from build123d import *

# Parameters (mm, degrees)
SKETCH1_R           = 3
BOSS_EXTRUDE1_DEPTH = 1
SKETCH4_R           = 1.5
CUT_EXTRUDE1_DEPTH  = 5.5


with BuildPart() as part:
    # Sketch1 → Boss-Extrude1 (new body)
    with BuildSketch(Plane(origin=(0, 0, 0), x_dir=(1, 0, 0), z_dir=(0, 1, 0))):
        with Locations(Location((0, 0, 0), (0, 0, 270))):
            Circle(SKETCH1_R)
    extrude(amount=BOSS_EXTRUDE1_DEPTH)

    # Sketch3 → Revolve2 (revolve)
    with BuildSketch(Plane(origin=(0, 0, 0), x_dir=(0, 0, -1), z_dir=(1, 0, 0))):
        with BuildLine():
            Line((-1.156919819, 1), (0, 1))
            Line((0, 1), (0, 4))
            Line((0, 4), (0, 7))
            ThreePointArc((0, 7), (-2.121320344, 6.121320344), (-3, 4))
            ThreePointArc((-3, 4), (-2.823253346, 2.98548507), (-2.313839638, 2.090511553))
            Line((-2.313839638, 2.090511553), (-2.313839638, 1))
            Line((-2.313839638, 1), (-1.156919819, 1))
        make_face()
    revolve(axis=Axis((0, 4, 0), (0, 1, 0)))

    # Sketch4 → Cut-Extrude1 (cut)
    with BuildSketch(Plane.XZ):
        with Locations(Location((0, 0, 0), (0, 0, 270))):
            Circle(SKETCH4_R)
    extrude(amount=-CUT_EXTRUDE1_DEPTH, mode=Mode.SUBTRACT)


solid = part.part
Geometry check sheet. Reference: the model listing, model coordinates, mm. A direction names the side the tool comes from. Coordinates: 2 decimals unless noted, no trailing zeros. Order: outer loops, then holes, each group sorted by start corner. A loop starts at its lowest first (then second) coordinate and runs counter-clockwise, first axis right, second up. Notation, with made-up numbers: (39, 18) - (85, 18) arc R21 cw to (85, 56) - close; hole circle Ø7 at (-6, 88). An arc over 180 degrees is marked (long way). Answer in a Markdown table with one row per item. Add a question column.
1) Cross-section at A-A, the plane z = 0. Record the cut outline in (x, y), then the cut area to 3 significant figures.
2) Set-up check for faces 4 (the cylindrical face through (0.45, 2.71, -1.43)), 5 (the flat face through (-2, 1, 2)): record each of +Z, -Z, +X, -X, +Y, -Y from which the full face is reachable in a straight line by a thin tool's end or side.
3) Release check for a two-part mould opening along Y. For faces 1 (the cylindrical face through (0.9, 0.49, 2.86)), 2 (the flat face through (-1.3, 0, 1.3)), 3 (the cylindrical face through (-2.26, 1.54, -0.5)) record: +Y half, -Y half, draft (parallel to the pull), parting line (faces both ways), or undercut.
4) Cross-section at B-B, the plane x = 0. Record the cut outline in (y, z).
5) Cross-section at D-D, the plane y = 4.5. Record the cut outline in (x, z), then the cut area to 3 significant figures.
6) Gauge pin test, flat ends, axial feed: P1, Ø2, axis at x = 1, z = -0.5, coming from the +Y side; P2, Ø0.9, axis at x = 0, z = -0.5, coming from the -Y side; P3, Ø1, axis at y = 3.5, z = -2, coming from the -X side. Record the tip position at first contact, or that the pin passes through.
7) Material ranges on line 1 along X through (y, z) = (1.7, 0); line 2 along X through (y, z) = (0.5, 1.25); line 3 along Y through (x, z) = (1.65, 2.25), recorded low to high. Write a range as [from, to].
8) Cross-section at C-C, the plane x = -2.55. Record the cut outline in (y, z), then the cut area to 3 significant figures.
Check result:
| question | item | result |
|---|---|---|
| 1 | outline | (-3, 0) - (-1.5, 0) - (-1.5, 5.5) - (1.5, 5.5) - (1.5, 0) - (3, 0) - (3, 1) - (2.31, 1) - (2.31, 2.09) arc R3 ccw (long way) to (-2.31, 2.09) - (-2.31, 1) - (-3, 1) - close |
| 1 | area | 19.3 mm² |
| 2 | face 4 | -Y |
| 2 | face 5 | none |
| 3 | face 1 | draft |
| 3 | face 2 | -Y half |
| 3 | face 3 | undercut |
| 4 | outline | (0, -3) - (1, -3) - (1, -2.31) - (2.09, -2.31) arc R3 ccw (long way) to (2.09, 2.31) - (1, 2.31) - (1, 3) - (0, 3) - (0, 1.5) - (5.5, 1.5) - (5.5, -1.5) - (0, -1.5) - close |
| 5 | outline | circle Ø5.92 at (0, 0); hole circle Ø3 at (0, 0) |
| 5 | area | 20.4 mm² |
| 6 | P1 | stops at y = 7 |
| 6 | P2 | stops at y = 5.5 |
| 6 | P3 | stops at x = -2.56 |
| 7 | line 1 | x = [-2.31, -1.5], [1.5, 2.31] |
| 7 | line 2 | x = [-2.73, -0.83], [0.83, 2.73] |
| 7 | line 3 | y = [0, 1], [2.9, 5.1] |
| 8 | outline | (0, -1.58) - (1, -1.58) - (1, 1.58) - (0, 1.58) - close; circle Ø3.16 at (4, 0) |
| 8 | area | 11.0 mm² |
